Design review of the part shown in the three views and the two pictorial views. Dimensions are in mm from the part's minimum x, y and z. A direction names the side the tool comes from. Give positions to 0.01 mm unless a question says otherwise; leave off trailing zeros. Write each loop counter-clockwise with the first axis right and the second up, starting at its lowest first coordinate (ties: lowest second). Pieces come first, ordered by that corner, then holes.
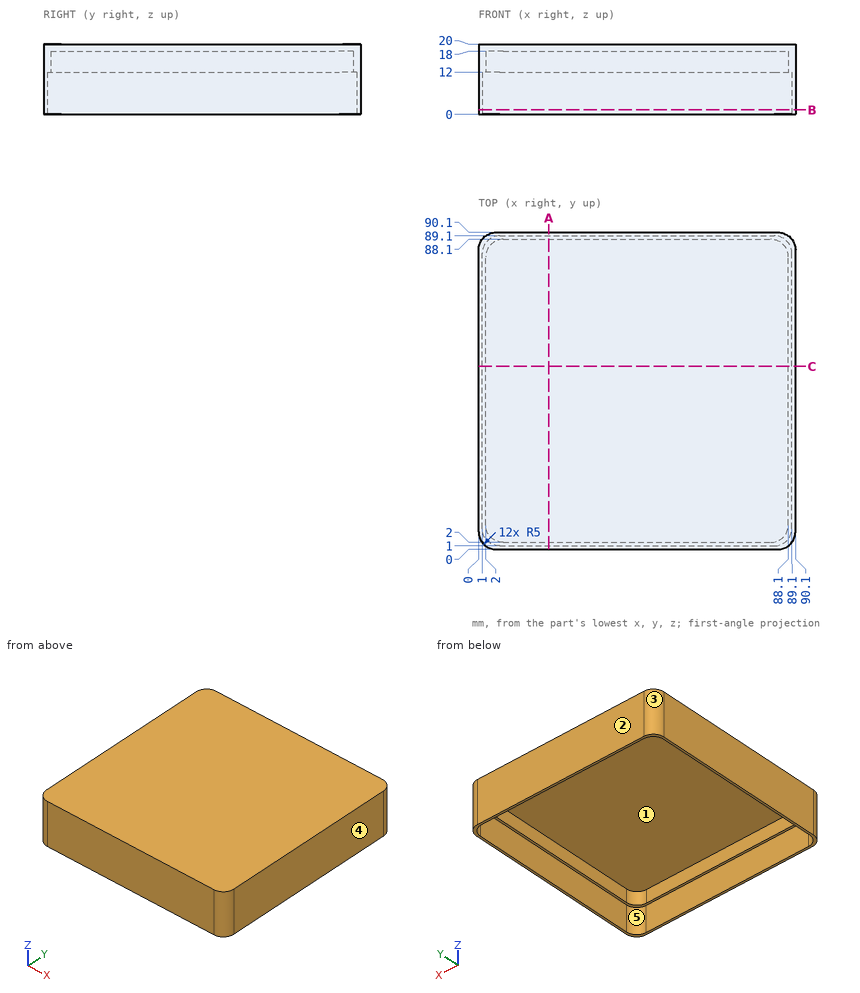
(1) Clearance check with a flat-ended pin moving along its axis: P1, Ø4, axis at x = 73, y = 51.5, coming from the -Z side. State where the tip first meets the part, or that it passes through.
Resolved:
P1: stops at z = 18
(2) Mouldability with a two-part tool opening along Y and no side actions: class the marked faces 3, 4 and 5 as pulls with the +Y half, pulls with the -Y half, needs draft (parallel to the pull), parting line crosses it, or undercut.
Resolved:
face 3: pulls with the +Y half
face 4: needs draft
face 5: undercut
(3) Tool access review of the marked faces 1 and 2: name each direction out of +Z, -Z, +X, -X, +Y, -Y from which nothing blocks a thin tool from reaching the whole face with its end or side.
Resolved:
face 1: -Z
face 2: +Z, -Z, +X, -X, +Y
(4) Consider section A-A, the plane x = 20. Give the boundary of the cut face in (y, z), then the cut area to 3 significant figures.
Resolved:
outline: (0, 0) - (1, 0) - (1, 12) - (2, 12) - (2, 18) - (88.1, 18) - (88.1, 12) - (89.1, 12) - (89.1, 0) - (90.1, 0) - (90.1, 20) - (0, 20) - close
area: 228 mm2
(5) To check wall thickness, follow L1, parallel to Y at x = 29, z = 15.5; L2, parallel to Y at x = 13, z = 2.25. State the ranges of each line that lie inside material, in increasing order.
Resolved:
L1: y = 0 to 2, 88.1 to 90.1
L2: y = 0 to 1, 89.1 to 90.1
(6) Consider section B-B, the plane z = 1.25. Give the boundary of the cut face in (x, y).
Resolved:
outline: (0, 5) arc R5 ccw to (5, 0) - (85.1, 0) arc R5 ccw to (90.1, 5) - (90.1, 85.1) arc R5 ccw to (85.1, 90.1) - (5, 90.1) arc R5 ccw to (0, 85.1) - close; hole (1, 6) arc R5 ccw to (6, 1) - (84.1, 1) arc R5 ccw to (89.1, 6) - (89.1, 84.1) arc R5 ccw to (84.1, 89.1) - (6, 89.1) arc R5 ccw to (1, 84.1) - close
